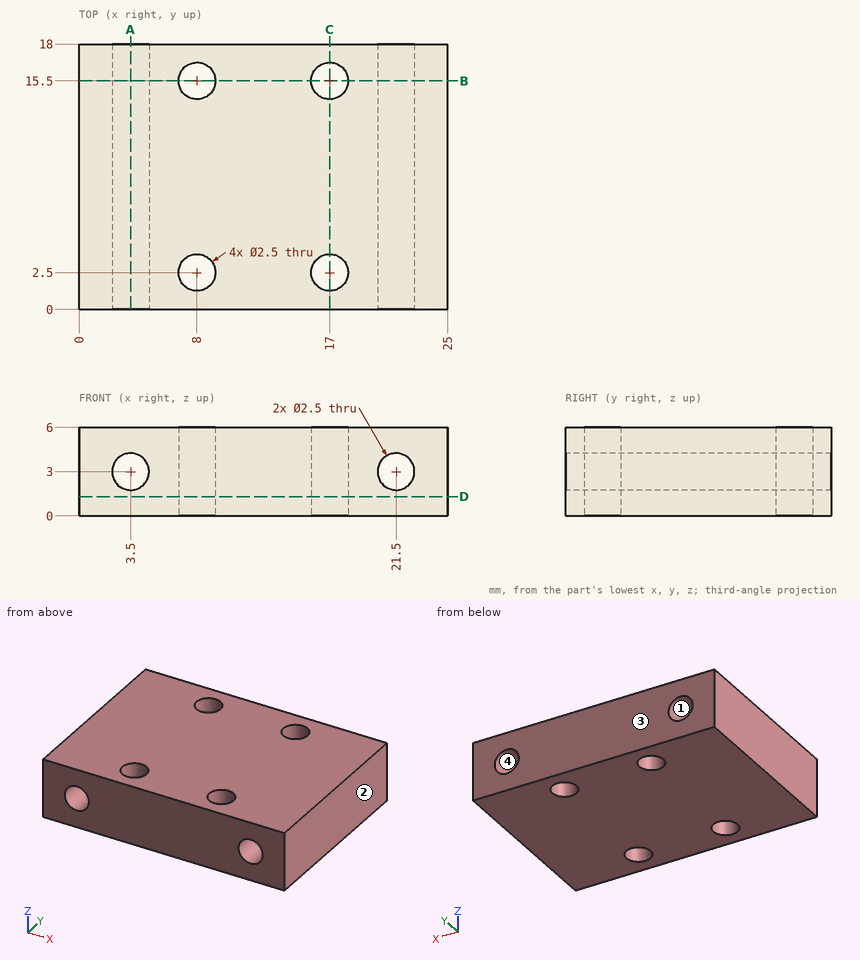
Design review of the part shown in the three views and the two pictorial views. Dimensions are in mm from the part's minimum x, y and z. Round coordinates to 2 decimals unless told otherwise and drop trailing zeros. Loops run counter-clockwise (first coordinate to the right, second up) from the corner with the lowest first, then second, coordinate; pieces in that order, holes last. Notation, with made-up numbers: (-3, 45.25) - (16, 45.25) arc R32 ccw to (16, 83.25) - close; hole circle Ø1 at (15, -4). An arc over 180 degrees is marked (long way). Write each question's results on one line, items separated by ' | '. Start each with the question number.
Q1. Draft analysis for pull direction X (two halves, no side actions). For the marked faces 1, 2, 3 and 4, state which applies: pulls with the +X half, pulls with the -X half, needs draft (parallel to the pull), parting line crosses it, or undercut.
Q2. Take a section at A-A on x = 3.5. Give the boundary of the cut face in (y, z), plus the area to 3 significant figures.
Q3. Take a section at D-D on z = 1.3. Give the boundary of the cut face in (x, y), plus the area to 3 significant figures.
Q4. Wall thickness on line 1 along Y through (x, z) = (8, 1.9); line 2 along X through (y, z) = (6.75, 2.7); line 3 along X through (y, z) = (14.5, 3.75): over which ranges is each line inside the solid? List them lowest first. Write a range as [from, to].
Q5. Insertion check: P1, Ø1.5, axis at x = 17, y = 2.5, coming from the +Z side. The pin has a flat end and moves straight along its axis. Give the tip position at first contact, or say it passes through.
Q6. Take a section at C-C on x = 17. Give the boundary of the cut face in (y, z).
Q7. Take a section at B-B on y = 15.5. Give the boundary of the cut face in (x, z).
Data:
1) face 1: undercut | face 2: pulls with the +X half | face 3: needs draft | face 4: undercut
2) outline: (0, 0) - (18, 0) - (18, 1.75) - (0, 1.75) - close; (0, 4.25) - (18, 4.25) - (18, 6) - (0, 6) - close | area: 63.0 mm²
3) outline: (0, 0) - (25, 0) - (25, 18) - (0, 18) - close; hole circle Ø2.5 at (8, 2.5); hole circle Ø2.5 at (8, 15.5); hole circle Ø2.5 at (17, 2.5); hole circle Ø2.5 at (17, 15.5) | area: 430 mm²
4) line 1: y = [0, 1.25], [3.75, 14.25], [16.75, 18] | line 2: x = [0, 2.29], [4.71, 20.29], [22.71, 25] | line 3: x = [0, 2.5], [4.5, 7.25], [8.75, 16.25], [17.75, 20.5], [22.5, 25]
5) P1: passes through
6) outline: (0, 0) - (1.25, 0) - (1.25, 6) - (0, 6) - close; (3.75, 0) - (14.25, 0) - (14.25, 6) - (3.75, 6) - close; (16.75, 0) - (18, 0) - (18, 6) - (16.75, 6) - close
7) outline: (0, 0) - (6.75, 0) - (6.75, 6) - (0, 6) - close; (9.25, 0) - (15.75, 0) - (15.75, 6) - (9.25, 6) - close; (18.25, 0) - (25, 0) - (25, 6) - (18.25, 6) - close; hole circle Ø2.5 at (3.5, 3); hole circle Ø2.5 at (21.5, 3)
